Design review of the part built by this model. Coordinates are the model's own, in mm. A direction names the side the tool comes from. Coordinates: 2 decimals unless noted, no trailing zeros. Loops run counter-clockwise (first coordinate to the right, second up) from the corner with the lowest first, then second, coordinate; pieces in that order, holes last. Notation, with made-up numbers: (5.25, 86.5) -> (21.25, 86.5) arc R21 cw to (21.25, 116.5) -> close; hole circle Ø2 at (82.25, 2). An arc over 180 degrees is marked (long way). Answer as a JSON object with one key per item and string values.
```python
from build123d import *

# Parameters (mm, degrees)
EXTRUDE028_DEPTH        = 15
BODY011_PLACEMENT_ANGLE = 30
BOX002_W                = 10
BOX002_H                = 10
BOX002_DEPTH            = 10


with BuildPart() as body011:
    # Sketch031 (on Cut) → Extrude028 (new body)
    with BuildSketch(Plane.XZ):
        Polygon((0, 3), (1, 4), (10, 4), (10, 9), (0, 9), align=None)
    extrude(amount=EXTRUDE028_DEPTH)


with BuildPart() as body011_1:
    # Body011 placement: moved
    add(body011.part.moved(Location((12, -8.6, 32.4))).rotate(Axis((12, -8.6, 32.4), (1, 0, 0)), BODY011_PLACEMENT_ANGLE))


with BuildPart() as cable:
    # Box002 → Box002 (new body)
    with BuildSketch(Plane(origin=(12, -19, 35), x_dir=(1, 0, 0), z_dir=(0, 1, 0))):
        with Locations((5, 5)):
            Rectangle(BOX002_W, BOX002_H)
    extrude(amount=BOX002_DEPTH)

    # Common: intersect Body011
    add(body011_1.part, mode=Mode.INTERSECT)


solid = cable.part
```
1) Add section B-B, the plane z = 34.2. Give the boundary of the cut face in (x, y).
Completed:
{"outline": "(12, -19) -> (22, -19) -> (22, -13.48) -> (13, -13.48) -> (12, -11.48) -> close"}
2) For faces 1 (the flat face through (17.437, -15.5, 33.035)), 2 (the flat face through (17, -19, 33)), list the 3-axis set-ups (+Z, -Z, +X, -X, +Y, -Y) from which the entire face can be reached by the end or side of a thin tool; tool diameter is ignored.
Completed:
{"face 1": "-Z, +X, +Y", "face 2": "+Z, -Z, +X, -X, -Y"}
3) Add section A-A, the plane y = -16. Give the boundary of the cut face in (x, z).
Completed:
{"outline": "(12, 31.59) -> (13, 32.75) -> (22, 32.75) -> (22, 35) -> (12, 35) -> close"}
4) Add section C-C, the plane x = 15.75. Give the boundary of the cut face in (y, z).
Completed:
{"outline": "(-19, 31.01) -> (-12.1, 35) -> (-19, 35) -> close"}
5) Clearance check with flat-ended pins moving along their axes: pin 1 Ø1.5 at (x, z) = (17, 33) entering from +Y; pin 2 Ø3 at (x, y) = (19.5, -11) entering from -Z; pin 3 Ø1 at (x, y) = (15.5, -12.5) entering from -Z; pin 4 Ø3 at (y, z) = (-12, 30.5) entering from +X. State where each tip first meets the part, or that it passes through.
Completed:
{"pin 1": "y = -14.26", "pin 2": "z = 34.77", "pin 3": "z = 34.48", "pin 4": "through"}
6) Wall thickness on probe 1 along X at (y, z) = (-15.25, 33); probe 2 along X at (y, z) = (-16, 31.9); probe 3 along Z at (x, y) = (16.25, -16.5): over which ranges is each line inside the solid? List them lowest first.
Completed:
{"probe 1": "12 to 12.84", "probe 2": "12 to 12.27", "probe 3": "32.46 to 35"}
7) Add section D-D, the plane z = 30.55. Give the boundary of the cut face in (x, y).
Completed:
{"outline": "(12, -19) -> (12.6, -19) -> (12, -17.8) -> close"}
